from build123d import *

# Parameters (mm, degrees)
MASTER_SKETCH_R       = 52.451
MASTER_SKETCH_R_2     = 9.525
MASTER_SKETCH_R_3     = 45.974
MASTER_SKETCH_R_4     = 27.4955
MASTER_SKETCH_R_5     = 6.5
BOSS_EXTRUDE2_DEPTH   = 3.048
F_5_0MM_DOWEL_HOLE1_D = 5
CIRPATTERN4_COUNT     = 4
M6_CLEARANCE_HOLE4_D  = 6.6
M8_CLEARANCE_HOLE1_D  = 9
CIRPATTERN3_COUNT     = 18
CUT_EXTRUDE2_DEPTH    = 284.854467488
CUT_EXTRUDE4_DEPTH    = 284.854467488
FILLET1_R             = 3.175


with BuildPart() as part:
    # Master Sketch → Boss-Extrude2 (new, symmetric)
    # profile 1 of 5: a face of its own
    with BuildSketch(Plane(origin=(0, 0, 0), x_dir=(1, 0, 0), z_dir=(0, 1, 0))):
        with BuildLine():
            ThreePointArc((-8.636, 127), (-36.396097826, 84.787887478), (-86.152093601, 93.552952189))
            Line((-86.152093601, 93.552952189), (-6.534964144, 18.470363023))
            ThreePointArc((-6.534964144, 18.470363023), (-3.773598517, 34.145603423), (9.525, 25.4))
            ThreePointArc((9.525, 25.4), (8.799952547, 21.754940307), (6.735192091, 18.664807909))
            Line((6.735192091, 18.664807909), (34.255961574, 46.185577392))
            ThreePointArc((34.255961574, 46.185577392), (59.945142207, 60.02346539), (89.010077776, 57.44457682))
            Line((89.010077776, 57.44457682), (207.987004211, 9.951947906))
            ThreePointArc((207.987004211, 9.951947906), (204.851852042, 25.601533276), (220.43444462, 22.148779315))
            Line((220.43444462, 22.148779315), (189.133864847, 105.44289655))
            ThreePointArc((189.133864847, 105.44289655), (188.207777178, 115.4635324), (192.51641215, 124.557840832))
            Line((192.51641215, 124.557840832), (212.800120602, 148.168522003))
            ThreePointArc((212.800120602, 148.168522003), (196.940842995, 150.353698677), (205.472725722, 163.899866417))
            Line((205.472725722, 163.899866417), (169.599038165, 163.514054819))
            ThreePointArc((169.599038165, 163.514054819), (163.800537316, 164.352688386), (158.531122559, 166.913779261))
            ThreePointArc((158.531122559, 166.913779261), (141.706259737, 175.147152322), (123.19, 177.9778))
            Line((123.19, 177.9778), (-54.61, 172.974))
            ThreePointArc((-54.61, 172.974), (-22.101472842, 159.508527158), (-8.636, 127))
        make_face()
        with Locations(Location((123.19, 116.0018, 0), (0, 0, 90))):
            Circle(MASTER_SKETCH_R, mode=Mode.SUBTRACT)
    # profile 2 of 5: a face of its own
    with BuildSketch(Plane(origin=(0, 0, 0), x_dir=(1, 0, 0), z_dir=(0, 1, 0))):
        with Locations((0, 25.4)):
            Circle(MASTER_SKETCH_R_2)
    # profile 3 of 5: a face of its own
    with BuildSketch(Plane(origin=(0, 0, 0), x_dir=(1, 0, 0), z_dir=(0, 1, 0))):
        with Locations((211.518208908, 18.79820239)):
            Circle(MASTER_SKETCH_R_2)
    # profile 4 of 5: a face of its own
    with BuildSketch(Plane(origin=(0, 0, 0), x_dir=(1, 0, 0), z_dir=(0, 1, 0))):
        with Locations((205.575158542, 154.375417219)):
            Circle(MASTER_SKETCH_R_2)
    # profile 5 of 5: a face of its own
    with BuildSketch(Plane(origin=(0, 0, 0), x_dir=(1, 0, 0), z_dir=(0, 1, 0))):
        with Locations((-54.61, 127)):
            Circle(MASTER_SKETCH_R_3)
        with Locations(Location((-54.61, 127, 0), (0, 0, 90))):
            Circle(MASTER_SKETCH_R_4, mode=Mode.SUBTRACT)
        with Locations(Location((-41.27121441, 90.351987789, 0), (0, 0, 90))):
            Circle(MASTER_SKETCH_R_5, mode=Mode.SUBTRACT)
        with Locations(Location((-67.94878559, 90.351987789, 0), (0, 0, 90))):
            Circle(MASTER_SKETCH_R_5, mode=Mode.SUBTRACT)
    extrude(amount=BOSS_EXTRUDE2_DEPTH, both=True)

    # Ø5.0mm Dowel Hole1 (through all)
    with Locations(Plane(origin=(0, 3.048, 0), x_dir=(1, 0, 0), z_dir=(0, 1, 0))):
        with Locations((123.19, 173.1518)):
            f_5_0mm_dowel_hole1 = Hole(F_5_0MM_DOWEL_HOLE1_D / 2)

    # CirPattern4: Ø5.0mm Dowel Hole1 ×4 about axis
    cirpattern4_axis = Axis((123.19, 0, -116.0018), (0, 1, 0))
    for i in range(1, CIRPATTERN4_COUNT):
        add(f_5_0mm_dowel_hole1.rotate(cirpattern4_axis, i * 360 / CIRPATTERN4_COUNT), mode=Mode.SUBTRACT)

    # M6 Clearance Hole4 (through all)
    with Locations(Plane(origin=(0, 3.048, 0), x_dir=(1, 0, 0), z_dir=(0, 1, 0))):
        with Locations((205.575158542, 154.375417219), (211.518208908, 18.79820239), (0, 25.4)):
            Hole(M6_CLEARANCE_HOLE4_D / 2)

    # M8 Clearance Hole1 (through all)
    with Locations(Plane(origin=(0, 3.048, 0), x_dir=(1, 0, 0), z_dir=(0, 1, 0))):
        with Locations((-54.61, 166)):
            m8_clearance_hole1 = Hole(M8_CLEARANCE_HOLE1_D / 2)

    # CirPattern3: M8 Clearance Hole1 ×18 about axis, 10 skipped
    cirpattern3_axis = Axis((-54.61, 3.048, -127), (0, -1, 0))
    add([m8_clearance_hole1.rotate(cirpattern3_axis, i * 360 / CIRPATTERN3_COUNT) for i in range(1, CIRPATTERN3_COUNT) if i not in (1, 3, 5, 7, 8, 10, 11, 13, 15, 17)], mode=Mode.SUBTRACT)

    # Topology 3 → Cut-Extrude2 (cut, through all)
    with BuildSketch(Plane(origin=(0, 3.048, 0), x_dir=(1, 0, 0), z_dir=(0, 1, 0))):
        with BuildLine():
            Line((148.232551201, 44.060262413), (194.821264757, 25.463207079))
            ThreePointArc((194.821264757, 25.463207079), (203.319232726, 27.16564341), (205.194131764, 35.627233252))
            Line((205.194131764, 35.627233252), (188.900120968, 78.987300553))
            ThreePointArc((188.900120968, 78.987300553), (183.658143307, 83.064639882), (177.648151764, 80.239214699))
            ThreePointArc((177.648151764, 80.239214699), (164.735029841, 65.81551406), (148.153589294, 55.823132596))
            ThreePointArc((148.153589294, 55.823132596), (144.236830733, 49.915140022), (148.232551201, 44.060262413))
        make_face()
        with BuildLine():
            Line((188.044823271, 154.186883307), (181.870154841, 154.120476454))
            ThreePointArc((181.870154841, 154.120476454), (179.135815493, 152.500048502), (179.17593949, 149.321874737))
            ThreePointArc((179.17593949, 149.321874737), (182.248718341, 143.510354832), (184.720207534, 137.418764347))
            ThreePointArc((184.720207534, 137.418764347), (187.127250613, 135.343061567), (190.127076346, 136.393510988))
            Line((190.127076346, 136.393510988), (194.150985671, 141.077429629))
            ThreePointArc((194.150985671, 141.077429629), (195.32544691, 149.601274428), (188.044823271, 154.186883307))
        make_face()
        with BuildLine():
            Line((14.548312592, 39.948312592), (27.520769483, 52.920769483))
            ThreePointArc((27.520769483, 52.920769483), (42.409632623, 63.819008448), (59.896219631, 69.707058463))
            ThreePointArc((59.896219631, 69.707058463), (66.885503662, 75.024623751), (66.553177874, 83.800508404))
            ThreePointArc((66.553177874, 83.800508404), (62.745475764, 91.688999032), (60.030376503, 100.016970919))
            ThreePointArc((60.030376503, 100.016970919), (55.6852269, 105.854731176), (48.48636159, 106.920614917))
            Line((48.48636159, 106.920614917), (0.801967439, 94.999516379))
            ThreePointArc((0.801967439, 94.999516379), (-0.72650755, 94.715480161), (-2.278234999, 94.620326131))
            Line((-2.278234999, 94.620326131), (-8.213826069, 94.620326131))
            ThreePointArc((-8.213826069, 94.620326131), (-12.770471536, 93.774733838), (-16.720335226, 91.350559531))
            Line((-16.720335226, 91.350559531), (-33.299725858, 74.771168898))
            ThreePointArc((-33.299725858, 74.771168898), (-37.018106584, 65.604842248), (-33.032755262, 56.551396808))
            Line((-33.032755262, 56.551396808), (-14.968322141, 39.515811377))
            ThreePointArc((-14.968322141, 39.515811377), (-10.208693563, 37.087360482), (-4.890365244, 37.60390848))
            ThreePointArc((-4.890365244, 37.60390848), (-0.192623775, 38.545871994), (4.530699747, 37.741953419))
            ThreePointArc((4.530699747, 37.741953419), (9.861879315, 37.381450483), (14.548312592, 39.948312592))
        make_face()
        with BuildLine():
            Line((60.61677272, 166.688039353), (-2.558763679, 164.910099257))
            ThreePointArc((-2.558763679, 164.910099257), (-10.543717082, 160.144406221), (-10.662758552, 150.846173049))
            ThreePointArc((-10.662758552, 150.846173049), (-6.896337856, 141.946787108), (-4.912213201, 132.489078911))
            ThreePointArc((-4.912213201, 132.489078911), (-0.884996506, 125.716198593), (6.865367013, 124.29414113))
            Line((6.865367013, 124.29414113), (55.673119377, 136.496079221))
            ThreePointArc((55.673119377, 136.496079221), (60.680188367, 139.024747182), (64.109569967, 143.463693382))
            ThreePointArc((64.109569967, 143.463693382), (66.313465528, 147.777775634), (68.831828447, 151.916170194))
            ThreePointArc((68.831828447, 151.916170194), (69.209050275, 161.796201373), (60.61677272, 166.688039353))
        make_face()
    extrude(amount=-CUT_EXTRUDE2_DEPTH, mode=Mode.SUBTRACT)

    # Sketch29 → Cut-Extrude4 (cut, through all)
    with BuildSketch(Plane(origin=(0, 3.048, 0), x_dir=(1, 0, 0), z_dir=(0, 1, 0))):
        with BuildLine():
            Line((-74.056787625, 92.575118721), (-76.882563864, 84.811362311))
            Line((-76.882563864, 84.811362311), (-66.583357956, 75.098740778))
            Line((-66.583357956, 75.098740778), (-61.840783555, 88.128856858))
            ThreePointArc((-61.840783555, 88.128856858), (-70.171916521, 84.243985754), (-74.056787625, 92.575118721))
        make_face()
    extrude(amount=-CUT_EXTRUDE4_DEPTH, mode=Mode.SUBTRACT)

    # Fillet1
    fillet1_edges = [part.edges().sort_by_distance(p)[0] for p in [
        (-66.583357956, 0, -75.098740778),
        (-76.882563864, 0, -84.811362311),
    ]]
    fillet(fillet1_edges, radius=FILLET1_R)


solid = part.part
Here's how the part is built. I have some questions about the finished solid (model axes, mm). A direction names the side the tool comes from. Round coordinates to 2 decimals unless told otherwise and drop trailing zeros. Order: outer loops, then holes, each group sorted by start corner. A loop starts at its lowest first (then second) coordinate and runs counter-clockwise, first axis right, second up. Notation, with made-up numbers: M 82,27.5 L 109,27.5 A26 cw 109,52.5 Z; hole C -4.5,45 d10. An arc over 180 degrees is marked long. Return JSON: item names as keys, results as strings. Group by question number.
1. If we section it at B-B on y = 2: State how many separate pieces and enclosed holes the cut face has, then the cut area to 3 significant figures.
2. On a 3-axis mill with a long thin cutter (end or side, diameter ignored), from which of +Z, -Z, +X, -X, +Y, -Y can I reach the whole of each face in a straight line? I mean faces 1 (the face through (60.619, 0.043, -138.975)), 2 (the face through (0.037, 0.043, -15.875)). Say none if no direction works.
3. Please list where these lines run through material, in increasing order: probe 1 along Z at (x, y) = (-21.5, -2.75); probe 2 along X at (y, z) = (-2, -141.5); probe 3 along Z at (x, y) = (23.5, 2.5).
4. I'm going to push flat-ended pins straight in: pin 1 Ø5.5 at (x, z) = (-54.61, -166) entering from +Y; pin 2 Ø6 at (x, z) = (123.19, -58.85) entering from -Y; pin 3 Ø3 at (y, z) = (1.5, -78.5) entering from -X. Where does each tip first touch, or does it pass through?
5. If we section it at A-A on x = 136: List the corners of the cut face in (y, z) for me.
6. If we mould it in two halves opening along X, with no side actions, what happens to faces 3 (the face through (-36.209, 0.043, -46.454)), 4 (the face through (188.183, -0.043, -115.323)), 5 (the face through (69.28, 0.04, -161.67))? For each: pulls with the +X half, pulls with the -X half, needs draft (parallel to the pull), parting line crosses it, or undercut.
Reply:
{
 "1": {"separate pieces": "1", "enclosed holes": "22", "area": "16,800 mm^2"},
 "2": {"face 1": "+Y, -Y", "face 2": "+Z, +Y, -Y"},
 "3": {"probe 1": "-173.91 to -111.95, -103.05 to -86.57, -45.68 to -32.58", "probe 2": "-98.24 to -77.97, -31.25 to -6.76, 62.97 to 77.35, 169.03 to 183.14, 194.49 to 207.07", "probe 3": "-175.17 to -165.64, -128.45 to -100.67, -48.9 to -35.43"},
 "4": {"pin 1": "through", "pin 2": "y = -3.05", "pin 3": "x = -65.89"},
 "5": {"outline": "M -3.05,-176.64 L 3.05,-176.64 L 3.05,-166.86 L -3.05,-166.86 Z; M -3.05,-65.14 L 3.05,-65.14 L 3.05,-38.69 L -3.05,-38.69 Z"},
 "6": {"face 3": "pulls with the -X half", "face 4": "pulls with the +X half", "face 5": "undercut"}
}
